Study the drawing (mm; zero at the part's minimum x, y, z) and answer. A direction names the side the tool comes from. Give positions to 0.01 mm unless a question says otherwise; leave off trailing zeros. Order: outer loops, then holes, each group sorted by start corner. A loop starts at its lowest first (then second) coordinate and runs counter-clockwise, first axis right, second up. Notation, with made-up numbers: (77.25, -20.75) -> (124.25, -20.75) arc R35 cw to (124.25, 13.25) -> close; hole circle Ø1 at (13.5, -10.75). An arc over 180 degrees is marked (long way). Answer as CSV lines item,"result". Start each with the question number.
1. Find the intervals of material crossed by L1, parallel to X at y = 3.1, z = 8.5; L2, parallel to Y at x = 11.75, z = 2; L3, parallel to X at y = 0.7, z = 7.75 (1 decimal), in increasing order.
2. Flat-ended cylindrical pins translate along their axes: pin 1 (2 mm diameter, centred on x = 6.5, y = 3, fed in from -Z); pin 2 (2 mm diameter, centred on y = 2, z = 14.5, fed in from -X); pin 3 (1.3 mm diameter, centred on x = 8, z = 9.5, fed in from -Y). Find the tip coordinate at first contact, or state that the pin passes through.
3. For a pull along X with two mould halves and no side action, classify the marked faces 1, 2, 3 and 4 as released by +X, released by -X, zero draft, split by the parting line, or undercut.
4. A cutting plane is placed at A-A (x = 8.5). Give the vertices of the cut face in (y, z).
5. A cutting plane is placed at D-D (x = 5.25). Give the vertices of the cut face in (y, z) (1 decimal).
6. A cutting plane is placed at C-C (z = 8.5). Give the vertices of the cut face in (x, y).
7. For the marked faces 5 and 6, determine the directions among +Z, -Z, +X, -X, +Y, -Y from which every point of the face is accessible in a straight line to the end or side of a thin tool.
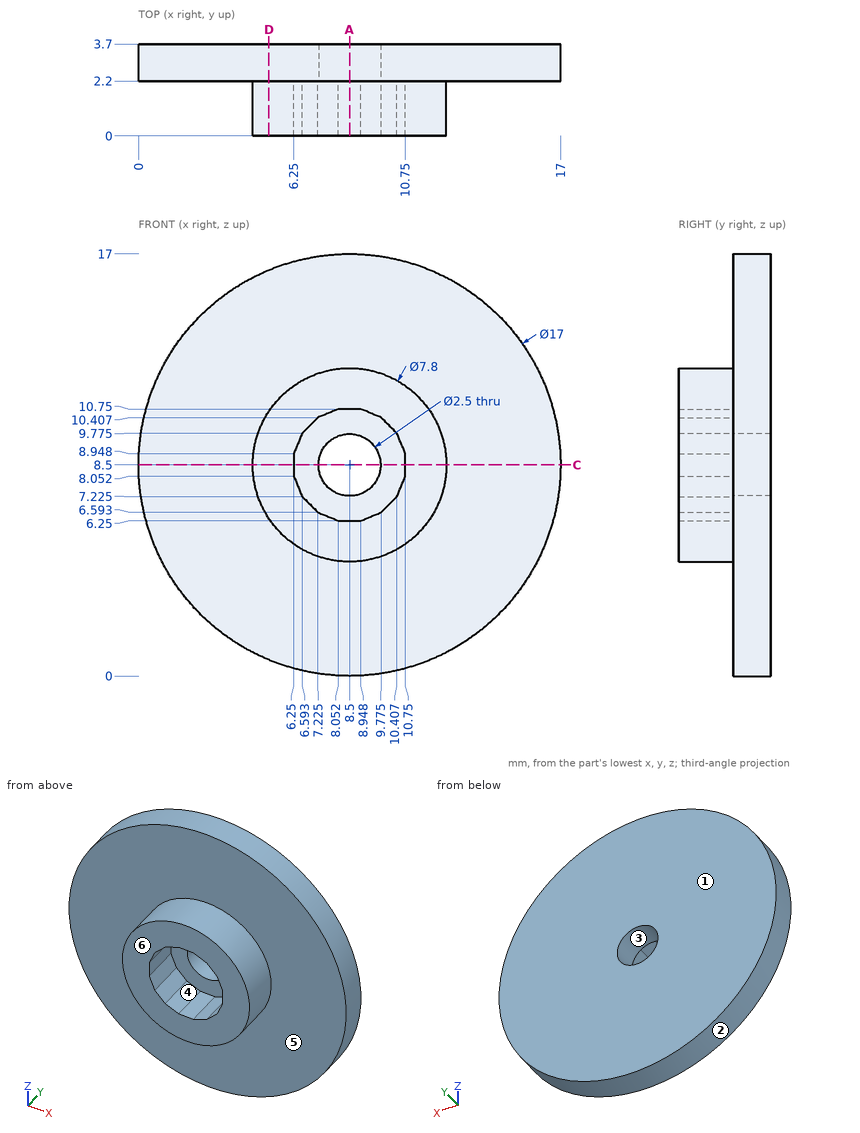
Answer sheet:
1,L1,"x = 0 to 7.25, 9.75 to 17"
1,L2,"y = 2.2 to 3.7"
1,L3,"x = 4.7 to 6.4, 10.6 to 12.3"
2,pin 1,"stops at z = 0.06"
2,pin 2,"stops at x = 1.64"
2,pin 3,"stops at y = 2.2"
3,face 1,"zero draft"
3,face 2,"split by the parting line"
3,face 3,"undercut"
3,face 4,"undercut"
4,outline,"(0, 4.6) -> (2.2, 4.6) -> (2.2, 0) -> (3.7, 0) -> (3.7, 7.25) -> (2.2, 7.25) -> (2.2, 6.25) -> (0, 6.25) -> close; (0, 10.75) -> (2.2, 10.75) -> (2.2, 9.75) -> (3.7, 9.75) -> (3.7, 17) -> (2.2, 17) -> (2.2, 12.4) -> (0, 12.4) -> close"
5,outline,"(0, 6.3) -> (2.2, 6.3) -> (2.2, 0.6) -> (3.7, 0.6) -> (3.7, 16.4) -> (2.2, 16.4) -> (2.2, 10.7) -> (0, 10.7) -> close"
6,outline,"(0, 2.2) -> (4.6, 2.2) -> (4.6, 0) -> (6.25, 0) -> (6.25, 2.2) -> (7.25, 2.2) -> (7.25, 3.7) -> (0, 3.7) -> close; (9.75, 2.2) -> (10.75, 2.2) -> (10.75, 0) -> (12.4, 0) -> (12.4, 2.2) -> (17, 2.2) -> (17, 3.7) -> (9.75, 3.7) -> close"
7,face 5,"-Y"
7,face 6,"+Z, -Z, +X, -X, -Y"
